Check sheet for the drawn part. Datum: minimum x, y, z corner. Units: mm. A direction names the side the tool comes from. Coordinates: 2 decimals unless noted, no trailing zeros. Write each loop counter-clockwise with the first axis right and the second up, starting at its lowest first coordinate (ties: lowest second). Pieces come first, ordered by that corner, then holes. Notation, with made-up numbers: (-7, 28) - (7, 28) arc R21 ccw to (7, 60) - close; hole circle Ø10 at (57, -11). An arc over 180 degrees is marked (long way). Answer as CSV lines item,"result". Start each with the question number.
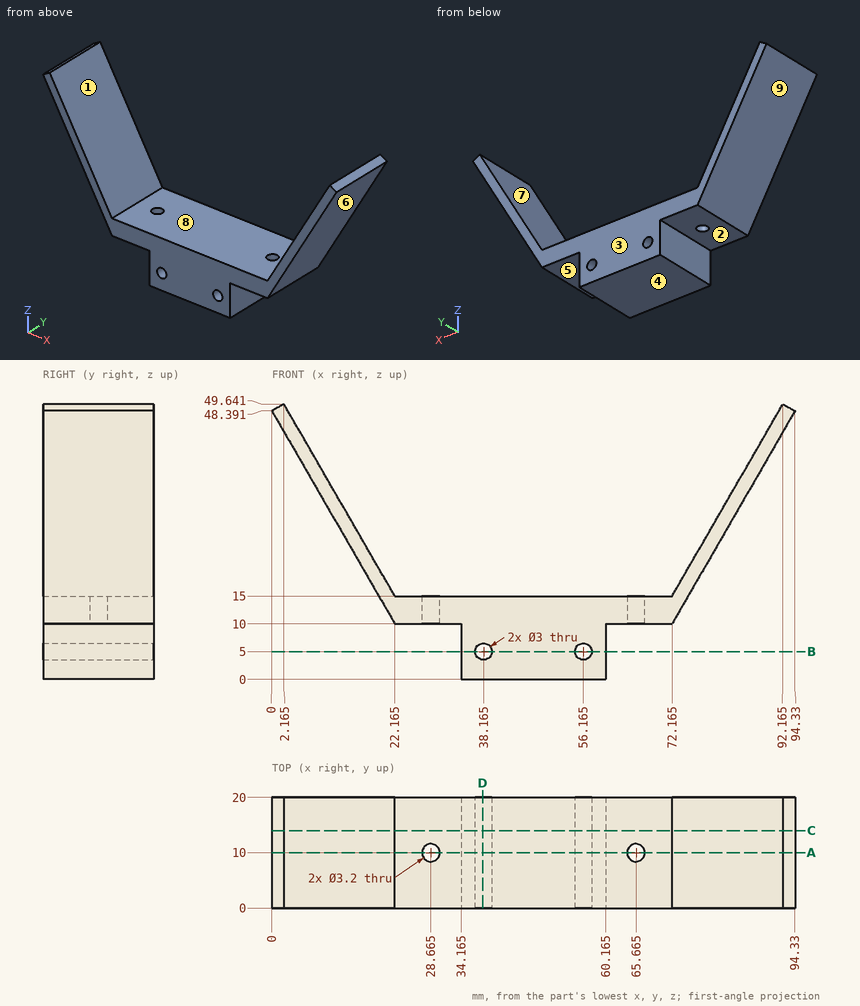
(1) Material ranges on probe 1 along X at (y, z) = (15, 5) (3 decimals); probe 2 along X at (y, z) = (16, 4) (1 decimal); probe 3 along X at (y, z) = (11, 39.5), recorded low to high. Write a range as from..to.
(2) Cross-section at D-D on x = 38. Record the boundary of the cut face in (y, z).
(3) Go/stop test with flat-tipped pins: P1, Ø1, axis at y = 9.5, z = 43, coming from the -X side; P2, Ø1, axis at y = 16, z = 44.5, coming from the +X side; P3, Ø10, axis at y = 3.5, z = 14, coming from the -X side. Record where each tip stops, or that it passes through.
(4) Cross-section at A-A on y = 10. Record the boundary of the cut face in (x, z) (3 decimals).
(5) Release check for a two-part mould opening along X. For the marked faces 6, 7, 8 and 9 record: pulls with the +X half, pulls with the -X half, needs draft (parallel to the pull), parting line crosses it, or undercut.
(6) Cross-section at C-C on y = 14. Record the boundary of the cut face in (x, z) (3 decimals).
(7) Cross-section at B-B on z = 5. Record the boundary of the cut face in (x, y) (3 decimals).
(8) Tool access check on the marked faces 1, 2, 3, 4 and 5. Record the directions out of +Z, -Z, +X, -X, +Y, -Y that give a thin tool (end or side, any length) a straight path to the whole face; none if there is none.
Checked values:
1,probe 1,"34.165..36.665, 39.665..54.665, 57.665..60.165"
1,probe 2,"34.2..37, 39.3..55, 57.3..60.2"
1,probe 3,"5.13..8.02, 86.31..89.2"
2,outline,"(0, 0) - (20, 0) - (20, 3.51) - (0, 3.51) - close; (0, 6.49) - (20, 6.49) - (20, 15) - (0, 15) - close"
3,P1,"x = 2.82"
3,P2,"x = 92.37"
3,P3,"x = 16.97"
4,outline,"(0, 48.391) - (22.165, 10) - (27.065, 10) - (27.065, 15) - (22.165, 15) - (2.165, 49.641) - close; (30.265, 10) - (34.165, 10) - (34.165, 0) - (60.165, 0) - (60.165, 10) - (64.065, 10) - (64.065, 15) - (30.265, 15) - close; (67.265, 10) - (72.165, 10) - (94.33, 48.391) - (92.165, 49.641) - (72.165, 15) - (67.265, 15) - close; hole circle Ø3 at (38.165, 5); hole circle Ø3 at (56.165, 5)"
5,face 6,"pulls with the +X half"
5,face 7,"undercut"
5,face 8,"undercut"
5,face 9,"pulls with the -X half"
6,outline,"(0, 48.391) - (22.165, 10) - (34.165, 10) - (34.165, 0) - (60.165, 0) - (60.165, 10) - (72.165, 10) - (94.33, 48.391) - (92.165, 49.641) - (72.165, 15) - (22.165, 15) - (2.165, 49.641) - close; hole circle Ø3 at (38.165, 5); hole circle Ø3 at (56.165, 5)"
7,outline,"(34.165, 0) - (36.665, 0) - (36.665, 20) - (34.165, 20) - close; (39.665, 0) - (54.665, 0) - (54.665, 20) - (39.665, 20) - close; (57.665, 0) - (60.165, 0) - (60.165, 20) - (57.665, 20) - close"
8,face 1,"+Z, +Y, -Y"
8,face 2,"-Z, -X, +Y, -Y"
8,face 3,"+Z, -Z, +X, -X, +Y"
8,face 4,"-Z, +X, -X, +Y, -Y"
8,face 5,"-Z, +X, +Y, -Y"
